```python
from build123d import *

# Parameters (mm, degrees)
SKETCH_1_W          = 200
SKETCH_1_H          = 240
SKETCH_1_R          = 13
EXTRUDE_323_DEPTH   = 8
SKETCH_2_W          = 8
SKETCH_2_H          = 240
EXTRUDE_1_DEPTH     = 92
SKETCH_3_R          = 13
CUT_EXTRUDE_1_DEPTH = 329.024389337
CHAMFER_1_SIZE      = 1


with BuildPart() as part:
    # 草图1 → Extrude 323 (new body)
    with BuildSketch(Plane.XY):
        with Locations((100, 120)):
            Rectangle(SKETCH_1_W, SKETCH_1_H)
        with Locations((160, 40)):
            Circle(SKETCH_1_R, mode=Mode.SUBTRACT)
        with Locations((160, 120)):
            Circle(SKETCH_1_R, mode=Mode.SUBTRACT)
        with Locations((160, 200)):
            Circle(SKETCH_1_R, mode=Mode.SUBTRACT)
    extrude(amount=EXTRUDE_323_DEPTH)

    # 草图2 → 凸台-拉伸1 (add)
    with BuildSketch(Plane.XY.offset(8)):
        with Locations((4, 120)):
            Rectangle(SKETCH_2_W, SKETCH_2_H)
    extrude(amount=EXTRUDE_1_DEPTH)

    # 草图3 → 切除-拉伸1 (cut, through all)
    with BuildSketch(Plane.ZY):
        with Locations((52, 200)):
            Circle(SKETCH_3_R)
        with Locations((52, 120)):
            Circle(SKETCH_3_R)
        with Locations((52, 40)):
            Circle(SKETCH_3_R)
    extrude(amount=-CUT_EXTRUDE_1_DEPTH, mode=Mode.SUBTRACT)

    # 倒角1
    chamfer_1_edges = [part.edges().sort_by_distance(p)[0] for p in [
        (200, 120, 8),
        (147, 40, 0),
        (147, 40, 8),
        (104, 240, 8),
        (147, 120, 0),
        (147, 120, 8),
        (147, 200, 0),
        (147, 200, 8),
        (104, 0, 8),
        (8, 120, 8),
        (8, 0, 54),
        (8, 240, 54),
        (0, 120, 100),
        (8, 120, 100),
        (8, 200, 39),
        (0, 200, 39),
        (100, 240, 0),
        (8, 120, 39),
        (0, 120, 39),
        (8, 40, 39),
        (0, 40, 39),
        (200, 120, 0),
        (100, 0, 0),
        (0, 120, 0),
        (0, 240, 50),
        (0, 0, 50),
    ]]
    chamfer(chamfer_1_edges, length=CHAMFER_1_SIZE)


solid = part.part
```
The model under review builds one solid part; all positions refer to its coordinate system, in mm. Round coordinates to 2 decimals unless told otherwise and drop trailing zeros. Write each loop counter-clockwise with the first axis right and the second up, starting at its lowest first coordinate (ties: lowest second). Pieces come first, ordered by that corner, then holes. Notation, with made-up numbers: (14.25, 5.25) - (28.25, 5.25) arc R11 cw to (28.25, 10.25) - close; hole circle Ø10 at (66.5, -28). An arc over 180 degrees is marked (long way). One line per question, with ' | ' between items.
Item 1: For P1, Ø1, axis at x = 113, y = 183.5, coming from the +Z side, flat-tipped, find the tip position at first contact; note if it passes through.
Resolved:
P1: stops at z = 8
Item 2: Add section D-D, the plane y = 71.5. Give the boundary of the cut face in (x, z), then the cut area to 3 significant figures.
Resolved:
outline: (0, 1) - (1, 0) - (199, 0) - (200, 1) - (200, 7) - (199, 8) - (9, 8) - (8, 9) - (8, 99) - (7, 100) - (1, 100) - (0, 99) - close | area: 2,330 mm2
Item 3: Add section A-A, the plane x = 160. State how many separate pieces and enclosed holes the cut face has, then the cut area to 3 significant figures.
Resolved:
separate pieces: 4 | enclosed holes: 0 | area: 1,290 mm2
Item 4: Add section C-C, the plane z = 86. Give the boundary of the cut face in (x, y), then the cut area to 3 significant figures.
Resolved:
outline: (0, 1) - (1, 0) - (7, 0) - (8, 1) - (8, 239) - (7, 240) - (1, 240) - (0, 239) - close | area: 1,920 mm2
Item 5: To check wall thickness, follow probe 1 along Y at (x, z) = (160, 5); probe 2 along Z at (x, y) = (42, 202). State the ranges of each line that lie inside material, in increasing order.
Resolved:
probe 1: y = 0 to 27, 53 to 107, 133 to 187, 213 to 240 | probe 2: z = 0 to 8
Item 6: The part is to be moulded in two halves that separate along X. For faces 1 (the face through (200, 118, 4)), 2 (the face through (71, 240, 6)), 3 (the face through (172.4, 43.9, 4)), say which applies: pulls with the +X half, pulls with the -X half, needs draft (parallel to the pull), parting line crosses it, or undercut.
Resolved:
face 1: pulls with the +X half | face 2: needs draft | face 3: undercut
Item 7: Add section B-B, the plane y = 120. Give the boundary of the cut face in (x, z).
Resolved:
outline: (0, 1) - (1, 0) - (146, 0) - (147, 1) - (147, 7) - (146, 8) - (9, 8) - (8, 9) - (8, 38) - (7, 39) - (1, 39) - (0, 38) - close; (0, 66) - (1, 65) - (7, 65) - (8, 66) - (8, 99) - (7, 100) - (1, 100) - (0, 99) - close; (173, 1) - (174, 0) - (199, 0) - (200, 1) - (200, 7) - (199, 8) - (174, 8) - (173, 7) - close
